Geometry check sheet. Reference: the model listing, model coordinates, mm. Face numbers are marked on the shaded views. A direction names the side the tool comes from. Round coordinates to 2 decimals unless told otherwise and drop trailing zeros. Loops run counter-clockwise (first coordinate to the right, second up) from the corner with the lowest first, then second, coordinate; pieces in that order, holes last.
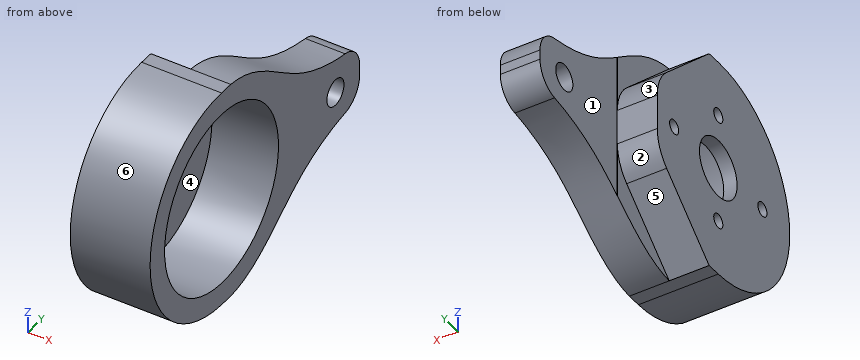
```python
from build123d import *

# Parameters (mm, degrees)
SKETCH1_R               = 10
SKETCH1_R_2             = 0.8
SKETCH1_R_3             = 3.301767793
BOSS_EXTRUDE1_DEPTH     = 1.5
SKETCH2_R               = 10
BOSS_EXTRUDE2_DEPTH     = 9
SKETCH3_R               = 1.5
CUT_EXTRUDE1_DEPTH      = 1
CUT_EXTRUDE1_DEPTH_BACK = 10
FILLET1_R               = 3
CUT_EXTRUDE2_DEPTH      = 10.565166147
CUT_EXTRUDE2_DEPTH_BACK = 16.531923841
CUT_EXTRUDE4_DEPTH      = 4.5
FILLET4_R               = 5


with BuildPart() as part:
    # Sketch1 → Boss-Extrude1 (new body)
    with BuildSketch(Plane(origin=(0, 0, 0), x_dir=(0, 0, -1), z_dir=(1, 0, 0))):
        with Locations((2.983378847, 10.826778074)):
            Circle(SKETCH1_R)
        with Locations((2.983378847, 18.576778074)):
            Circle(SKETCH1_R_2, mode=Mode.SUBTRACT)
        with Locations((2.983378847, 3.076778074)):
            Circle(SKETCH1_R_2, mode=Mode.SUBTRACT)
        with Locations((-3.266621153, 10.826778074)):
            Circle(SKETCH1_R_2, mode=Mode.SUBTRACT)
        with Locations((9.233378847, 10.826778074)):
            Circle(SKETCH1_R_2, mode=Mode.SUBTRACT)
        with Locations((2.983378847, 10.826778074)):
            Circle(SKETCH1_R_3, mode=Mode.SUBTRACT)
    extrude(amount=BOSS_EXTRUDE1_DEPTH)

    # Sketch2 → Boss-Extrude2 (add)
    with BuildSketch(Plane.ZY):
        with BuildLine():
            Line((-15.531923741, 35.094698666), (9.565166047, 35.094698666))
            Line((9.565166047, 35.094698666), (9.565166047, 10.826778074))
            ThreePointArc((9.565166047, 10.826778074), (-2.983378847, -1.721766821), (-15.531923741, 10.826778074))
            Line((-15.531923741, 10.826778074), (-15.531923741, 35.094698666))
        make_face()
        with Locations((-2.983378847, 10.826778074)):
            Circle(SKETCH2_R, mode=Mode.SUBTRACT)
    extrude(amount=-BOSS_EXTRUDE2_DEPTH)

    # Sketch3 → Cut-Extrude1 (cut, two sides)
    with BuildSketch(Plane(origin=(9, 0, 0), x_dir=(0, 0, -1), z_dir=(1, 0, 0))) as cut_extrude1_sk:
        with Locations((2.983378847, 30.826778074)):
            Circle(SKETCH3_R)
        with BuildLine():
            Line((-0.254346927, 36.150412664), (-0.254346927, 97.572569437))
            Line((-0.254346927, 97.572569437), (-16.389018159, 97.572569437))
            Line((-16.389018159, 97.572569437), (-16.389018159, 8.14109285))
            Line((-16.389018159, 8.14109285), (-9.565166047, 10.826778074))
            add(Edge.make_bspline(
                [(-9.565166047, 10.826778074), (-9.996776932, 16.621947073), (-2.416923511, 22.902398079), (-0.279431234, 32.151841163), (-0.254346927, 36.150412664)],
                knots=[0, 0, 0, 0, 0.563274164, 1, 1, 1, 1], degree=3))
        make_face()
        with BuildLine():
            Line((22.355775853, 8.14109285), (15.531923741, 10.826778074))
            add(Edge.make_bspline(
                [(15.531923741, 10.826778074), (15.963534626, 16.621947073), (8.383681205, 22.902398079), (6.246188928, 32.151841163), (6.221104621, 36.150412664)],
                knots=[0, 0, 0, 0, 0.563274164, 1, 1, 1, 1], degree=3))
            Line((6.221104621, 36.150412664), (6.221104621, 97.572569437))
            Line((6.221104621, 97.572569437), (22.355775853, 97.572569437))
            Line((22.355775853, 97.572569437), (22.355775853, 8.14109285))
        make_face()
    extrude(amount=CUT_EXTRUDE1_DEPTH, mode=Mode.SUBTRACT)
    extrude(cut_extrude1_sk.sketch, amount=-CUT_EXTRUDE1_DEPTH_BACK, mode=Mode.SUBTRACT)

    # Fillet1
    fillet1_edges = [part.edges().sort_by_distance(p)[0] for p in [
        (4.5, 35.094698666, -6.248898777),
        (4.5, 35.094698666, 0.282141083),
    ]]
    fillet(fillet1_edges, radius=FILLET1_R)

    # Sketch5 → Cut-Extrude2 (cut, two sides)
    with BuildSketch(Plane.XY) as cut_extrude2_sk:
        Polygon((4.519735145, 37.354194786), (-3.918381593, 39.378706192), (-3.918381593, 21.53545024), (4.519735145, 21.53545024), align=None)
    extrude(amount=CUT_EXTRUDE2_DEPTH, mode=Mode.SUBTRACT)
    extrude(cut_extrude2_sk.sketch, amount=-CUT_EXTRUDE2_DEPTH_BACK, mode=Mode.SUBTRACT)

    # Sketch6 → Cut-Extrude4 (cut)
    with BuildSketch(Plane.ZY):
        Polygon((-15.531923741, 12.43637897), (-7.23722927, 21.53545024), (-16.045201911, 21.53545024), align=None)
        Polygon((9.565166047, 12.43637897), (1.120335679, 21.53545024), (9.021007351, 21.981126747), (10.387134826, 13.199246596), align=None)
    extrude(amount=-CUT_EXTRUDE4_DEPTH, mode=Mode.SUBTRACT)

    # Fillet4
    fillet4_edges = [part.edges().sort_by_distance(p)[0] for p in [
        (2.25, 21.53545024, -7.23722927),
        (2.25, 21.53545024, 1.120335679),
    ]]
    fillet(fillet4_edges, radius=FILLET4_R)


solid = part.part
```
1) Mould release check, pull along Y, two halves, no side actions. Record for the marked faces 4, 5 and 6: +Y half, -Y half, draft (parallel to the pull), parting line (faces both ways), or undercut.
Report:
face 4: undercut
face 5: +Y half
face 6: -Y half
2) Scan lines: line 1 along X through (y, z) = (8.5, -8.5); line 2 along Z through (x, y) = (3.5, 16); line 3 along Y through (x, z) = (6.75, -4.25). Record each from-to range of solid material in increasing order.
Report:
line 1: x = 0 to 1.5
line 2: z = -12.28 to -11.54, 5.57 to 6.26
line 3: y = -1.66 to 0.91, 20.75 to 30.02, 31.63 to 35.01
3) Sectioned sample at C-C, the plane x = 6. State how many separate pieces and enclosed holes the cut face has, then the cut area to 3 significant figures.
Report:
separate pieces: 1
enclosed holes: 2
area: 296 mm2
4) Access from +Z, -Z, +X, -X, +Y, -Y to the whole of each face (thin tool, end or side, straight path). Record for the marked faces 1, 2 and 3.
Report:
face 1: +Z, -Z, -X, +Y
face 2: -Z, -X, +Y
face 3: +Z, -X, +Y
5) Gauge pin test, flat ends, axial feed: pin 1 (3 mm diameter, centred on y = 30, z = 3, fed in from -X); pin 2 (4 mm diameter, centred on y = 27.5, z = -4.5, fed in from -X); pin 3 (1.5 mm diameter, centred on x = 1.5, y = 3, fed in from +Z); pin 4 (1.5 mm diameter, centred on x = 2, z = -8, fed in from -Y). Record the tip position at first contact, or that the pin passes through.
Report:
pin 1: passes through
pin 2: stops at x = 4.52
pin 3: stops at z = 7.38
pin 4: stops at y = -0.97
6) Sectioned sample at A-A, the plane y = 12. Record the cut outline in (x, z), then the cut area to 3 significant figures.
Report:
outline: (0, -15.53) - (9, -15.53) - (9, -12.91) - (1.5, -12.91) - (1.5, -6.07) - (0, -6.07) - close; (0, 0.1) - (1.5, 0.1) - (1.5, 6.95) - (9, 6.95) - (9, 9.57) - (0, 9.57) - close
area: 67.7 mm2
7) Sectioned sample at B-B, the plane x = 2.5. Record the cut outline in (y, z), then the cut area to 3 significant figures.
Report:
outline: (10.83, -15.53) - (12.44, -15.53) - (19.9, -8.72) arc R5 ccw to (21.54, -5.03) - (21.54, -1.06) arc R5 ccw to (19.94, 2.6) - (12.44, 9.57) - (10.83, 9.57) arc R12.55 ccw to start; hole circle Ø20 at (10.83, -2.98)
area: 125 mm2
